from build123d import *

# Parameters (mm, degrees)
F0_W      = 106
F0_H      = 44
F1_DEPTH  = 47
F2_T      = -1.6
F3_W      = 47
F3_H      = 1.2
F3_W_2    = 46.578951
F4_DEPTH  = 42.4
F6_DEPTH  = 143
F7_W      = 11.8
F7_H      = 6
F8_DEPTH  = 7
F10_DEPTH = 5
F11_W     = 11.8
F11_H     = 6
F12_DEPTH = 7
F13_W     = 11.8
F13_H     = 6
F14_DEPTH = 7
F15_W     = 11.8
F15_H     = 6
F16_DEPTH = 7
F18_DEPTH = 119


with BuildPart() as f1:
    # F0 (on Right) → F1 (new body)
    with BuildSketch(Plane.YZ):
        Rectangle(F0_W, F0_H)
    extrude(amount=F1_DEPTH)

    # F2
    f2_openings = [f1.faces().sort_by_distance(p)[0] for p in [
        (23.5, 0, 22),
    ]]
    offset(amount=F2_T, openings=f2_openings)

    # F3 (on face) → F4 (join)
    with BuildSketch(Plane.XY.offset(-20.4)):
        with Locations((23.5, 0)):
            Rectangle(F3_W, F3_H)
        with Locations((23.289475, 13)):
            Rectangle(F3_W_2, F3_H)
        with Locations((23.289475, 26)):
            Rectangle(F3_W_2, F3_H)
        with Locations((23.289475, 39)):
            Rectangle(F3_W_2, F3_H)
        with Locations((23.289475, -13)):
            Rectangle(F3_W_2, F3_H)
        with Locations((23.289475, -26)):
            Rectangle(F3_W_2, F3_H)
        with Locations((23.289475, -39)):
            Rectangle(F3_W_2, F3_H)
    extrude(amount=F4_DEPTH)

    # F5 (on face) → F6 (cut)
    with BuildSketch(Plane(origin=(0, 53, 0), x_dir=(-1, 0, 0), z_dir=(0, 1, 0))):
        Polygon((-4.991917, 22), (-47, 22), (-47, -18.157896), align=None)
    extrude(amount=-F6_DEPTH, mode=Mode.SUBTRACT)

    # F7 (on face) → F8 (join)
    with BuildSketch(Plane.YZ.offset(1.6)):
        with Locations((32.5, 19)):
            Rectangle(F7_W, F7_H)
    extrude(amount=F8_DEPTH)

    # F9 (on face) → F10 (join)
    with BuildSketch(Plane(origin=(0, 0, 0), x_dir=(0, -1, 0), z_dir=(-1, 0, 0))):
        Polygon((-53, -22), (-8.871453, -22), (-3.871453, -22), (53, -22), (53, -10), (-53, -10), align=None)
    extrude(amount=F10_DEPTH)

    # F11 (on face) → F12 (join)
    with BuildSketch(Plane.YZ.offset(1.6)):
        with Locations((6.5, 19)):
            Rectangle(F11_W, F11_H)
    extrude(amount=F12_DEPTH)

    # F13 (on face) → F14 (join)
    with BuildSketch(Plane.YZ.offset(1.6)):
        with Locations((-19.5, 19)):
            Rectangle(F13_W, F13_H)
    extrude(amount=F14_DEPTH)

    # F15 (on face) → F16 (join)
    with BuildSketch(Plane.YZ.offset(1.6)):
        with Locations((-45.5, 19)):
            Rectangle(F15_W, F15_H)
    extrude(amount=F16_DEPTH)

    # F17 (on face) → F18 (cut)
    with BuildSketch(Plane(origin=(0, 53, 0), x_dir=(-1, 0, 0), z_dir=(0, 1, 0))):
        Polygon((5, -22), (5, -10), (0.393632, -22), align=None)
    extrude(amount=-F18_DEPTH, mode=Mode.SUBTRACT)


solid = f1.part
Check sheet for the modelled part. Datum: model origin and axes. Units: mm. A direction names the side the tool comes from. Give positions to 0.01 mm unless a question says otherwise; leave off trailing zeros. Write each loop counter-clockwise with the first axis right and the second up, starting at its lowest first coordinate (ties: lowest second). Pieces come first, ordered by that corner, then holes. Notation, with made-up numbers: (39.25, -6) -> (97.25, -6) arc R25 ccw to (97.25, 11) -> close; hole circle Ø4 at (-29.5, 87). An arc over 180 degrees is marked (long way). Write item = value, one per line.
Item 1: Sectioned sample at B-B on y = -19. Record the boundary of the cut face in (x, z).
Output:
outline = (-5, -10) -> (-0.39, -22) -> (47, -22) -> (47, -18.16) -> (45.4, -16.63) -> (45.4, -20.4) -> (1.6, -20.4) -> (1.6, 16) -> (8.6, 16) -> (8.6, 22) -> (0, 22) -> (0, -10) -> close
Item 2: Tool access check on faces 5 (the flat face through (-2.729, 0.742, -15.916)), 6 (the flat face through (5, 32, 16)), 7 (the flat face through (18, 13.6, -4)), 8 (the flat face through (8, -13.6, 21)), 9 (the flat face through (23, -46, -20.4)). Record the directions out of +Z, -Z, +X, -X, +Y, -Y that give a thin tool (end or side, any length) a straight path to the whole face; none if there is none.
Output:
face_5 = -Z, -X, +Y, -Y
face_6 = +X
face_7 = +Z
face_8 = +Z, +X
face_9 = none
Item 3: Release check for a two-part mould opening along Y. For faces 1 (the flat face through (8, 38.4, 21)), 2 (the flat face through (18, -25.4, -6)), 3 (the flat face through (0, 46, 6)), 4 (the flat face through (16, -53, -5)) record: +Y half, -Y half, draft (parallel to the pull), parting line (faces both ways), or undercut.
Output:
face_1 = +Y half
face_2 = undercut
face_3 = draft
face_4 = -Y half
Item 4: Scan lines: probe 1 along Z at (x, y) = (34, -36.5); probe 2 along X at (y, z) = (-23, 0); probe 3 along Z at (x, y) = (7, -43.5). Record each from-to range of solid material in increasing order. Write a range as from..to.
Output:
probe_1 = -22..-20.4
probe_2 = 0..1.6
probe_3 = -22..-20.4, 16..22
Item 5: Sectioned sample at A-A on y = -6. Record the boundary of the cut face in (x, z), and give its area (3 significant figures).
Output:
outline = (-5, -10) -> (-0.39, -22) -> (47, -22) -> (47, -18.16) -> (45.4, -16.63) -> (45.4, -20.4) -> (1.6, -20.4) -> (1.6, 22) -> (0, 22) -> (0, -10) -> close
area = 180 mm^2
Item 6: Gauge pin test, flat ends, axial feed: pin 1 (1.5 mm diameter, centred on x = 8.5, y = 41.5, fed in from +Z); pin 2 (3 mm diameter, centred on y = 7, z = -19.5, fed in from -X); pin 3 (6 mm diameter, centred on y = 9, z = -8.5, fed in from +X). Record the tip position at first contact, or that the pin passes through.
Output:
pin_1 = -20.4
pin_2 = -1.93
pin_3 = 1.6
